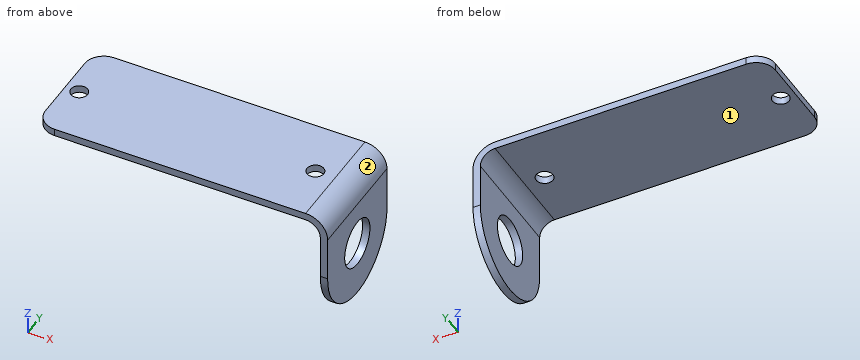
```python
from build123d import *

# Parameters (mm, degrees)
SKETCH1_W                  = 53.93
SKETCH1_H                  = 22.93
BOSS_EXTRUDE1_DEPTH        = 1.5
M3_CLEARANCE_HOLE1_D       = 3.4
M3_CLEARANCE_HOLE1_DEPTH   = 27
M3_CLEARANCE_HOLE1_TIP     = 1.021463052
FILLET1_R                  = 3.9
BOSS_EXTRUDE2_START        = -1.5
SKETCH4_R                  = 4.875
BOSS_EXTRUDE2_DEPTH        = 1.5
SKETCHED_START             = 32.144466887
SKETCHED_BEND1_OUTLINE_W   = 22.93
SKETCHED_BEND1_OUTLINE_H   = 1.5
SKETCHED_BEND1_DEPTH       = 23.855533113
SKETCHED_START_2           = 28.119756887
SKETCHED_BEND1_2_OUTLINE_R = 4.875
SKETCHED_BEND1_2_DEPTH     = 4.5
SKETCHED_START_3           = -11.465
SKETCHED_BEND1_3_DEPTH     = 22.93


with BuildPart() as part:
    # Sketch1 → Boss-Extrude1 (new body)
    with BuildSketch(Plane.XY.offset(1.5)):
        Rectangle(SKETCH1_W, SKETCH1_H)
    extrude(amount=-BOSS_EXTRUDE1_DEPTH)

    # M3 Clearance Hole1
    with Locations(Plane.XY.offset(1.5)):
        with Locations((-24.0755, 0), (24.0755, 0)):
            Hole(M3_CLEARANCE_HOLE1_D / 2, depth=M3_CLEARANCE_HOLE1_DEPTH)
            with Locations((0, 0, -(M3_CLEARANCE_HOLE1_DEPTH + M3_CLEARANCE_HOLE1_TIP / 2))):  # 118° drill point
                Cone(0, M3_CLEARANCE_HOLE1_D / 2, M3_CLEARANCE_HOLE1_TIP, mode=Mode.SUBTRACT)

    # Fillet1
    fillet1_edges = [part.edges().sort_by_distance(p)[0] for p in [
        (-26.965, -11.465, 0.75),
        (-26.965, 11.465, 0.75),
        (26.965, 11.465, 0.75),
        (26.965, -11.465, 0.75),
    ]]
    fillet(fillet1_edges, radius=FILLET1_R)

    # Sketch4 → Boss-Extrude2 (add)
    with BuildSketch(Plane.XY.offset(1.5).offset(BOSS_EXTRUDE2_START)):
        with BuildLine():
            Line((23.065, 11.465), (43.065, 11.465))
            ThreePointArc((43.065, 11.465), (54.53, 0), (43.065, -11.465))
            Line((43.065, -11.465), (23.065, -11.465))
            ThreePointArc((23.065, -11.465), (25.822716447, -10.322716447), (26.965, -7.565))
            Line((26.965, -7.565), (26.965, 7.565))
            ThreePointArc((26.965, 7.565), (25.822716447, 10.322716447), (23.065, 11.465))
        make_face()
        with Locations((43.065, 0)):
            Circle(SKETCH4_R, mode=Mode.SUBTRACT)
    extrude(amount=BOSS_EXTRUDE2_DEPTH)

    # Sketched Bend1: read off the stored shape, not the designer's step
    # Sketched Bend1 outline → Sketched Bend1 (cut)
    with BuildSketch(Plane.YZ.offset(SKETCHED_START)):
        with Locations((0, 0.75)):
            Rectangle(SKETCHED_BEND1_OUTLINE_W, SKETCHED_BEND1_OUTLINE_H)
    extrude(amount=SKETCHED_BEND1_DEPTH, mode=Mode.SUBTRACT)

    # Sketched Bend1 2 outline → Sketched Bend1 2 (add)
    with BuildSketch(Plane.YZ.offset(SKETCHED_START_2)):
        with BuildLine():
            Line((-11.465, 0), (-11.465, -12.054756887))
            ThreePointArc((-11.465, -12.054756887), (0, -23.519756887), (11.465, -12.054756887))
            Line((11.465, -12.054756887), (11.465, 0))
            Line((11.465, 0), (-11.465, 0))
        make_face()
        with Locations((0, -12.054756887)):
            Circle(SKETCHED_BEND1_2_OUTLINE_R, mode=Mode.SUBTRACT)
    extrude(amount=SKETCHED_BEND1_2_DEPTH)

    # Sketched Bend1 3 outline → Sketched Bend1 3 (cut)
    with BuildSketch(Plane(origin=(0, 0, 0), x_dir=(1, 0, 0), z_dir=(0, 1, 0)).offset(SKETCHED_START_3)):
        with BuildLine():
            ThreePointArc((28.119756887, 0), (30.241077231, 0.878679656), (31.119756887, 3))
            Line((31.119756887, 3), (31.119756887, 25))
            Line((31.119756887, 25), (28.119756887, 25))
            Line((28.119756887, 25), (28.119756887, 0))
        make_face()
        with BuildLine():
            Line((32.619756887, 0), (32.619756887, 3))
            ThreePointArc((32.619756887, 3), (31.301737402, -0.181980515), (28.119756887, -1.5))
            Line((28.119756887, -1.5), (27, -1.5))
            Line((27, -1.5), (27, -3))
            Line((27, -3), (32.144466887, -3))
            Line((32.144466887, -3), (32.144466887, 0))
            Line((32.144466887, 0), (32.619756887, 0))
        make_face()
    extrude(amount=SKETCHED_BEND1_3_DEPTH, mode=Mode.SUBTRACT)


solid = part.part
```
Can you work these out from the model? Positions are in its coordinate system, mm. Face numbers are marked on the shaded views. A direction names the side the tool comes from. Give positions to 0.01 mm unless a question says otherwise; leave off trailing zeros. Loops run counter-clockwise (first coordinate to the right, second up) from the corner with the lowest first, then second, coordinate; pieces in that order, holes last. Notation, with made-up numbers: M 57,34.5 L 111,34.5 A11 cw 111,40.5 Z; hole C 20,40.25 d11. An arc over 180 degrees is marked long. Answer in a Markdown table with one row per item.
1. Suppose I cut it at B-B on y = -2.25. Write out the boundary of the cut face in (x, z) (3 decimals).
Taken from the geometry:
| item | result |
|---|---|
| outline | M -26.965,0 L 28.12,0 A3 cw 31.12,-3 L 31.12,-7.73 L 32.62,-7.73 L 32.62,-3 A4.5 ccw 28.12,1.5 L -26.965,1.5 Z; M 31.12,-23.297 L 32.62,-23.297 L 32.62,-16.379 L 31.12,-16.379 Z |
2. Suppose I cut it at A-A on z = -15.75. Write out the boundary of the cut face in (x, y), plus the area to 3 significant figures.
Taken from the geometry:
| item | result |
|---|---|
| outline | M 31.12,-10.85 L 32.62,-10.85 L 32.62,-3.18 L 31.12,-3.18 Z; M 31.12,3.18 L 32.62,3.18 L 32.62,10.85 L 31.12,10.85 Z |
| area | 23.0 mm² |
3. For pin 1 Ø5 at (x, y) = (25, 3.5) entering from -Z; pin 2 Ø10.5 at (y, z) = (2, -17) entering from -X, each with a flat end and sliding along its axis, tell me the tip position at first contact or that it passes through.
Taken from the geometry:
| item | result |
|---|---|
| pin 1 | stops at z = 0 |
| pin 2 | stops at x = 31.12 |
4. If I drill on line 1 along Z through (x, y) = (11, 0.5); line 2 along X through (y, z) = (10.25, -3.5); line 3 along Z through (x, y) = (31.9, 0), over which ranges is the centre line in solid material (lowest first)?
Taken from the geometry:
| item | result |
|---|---|
| line 1 | z = 0 to 1.5 |
| line 2 | x = 31.12 to 32.62 |
| line 3 | z = -23.52 to -16.93, -7.18 to -0.56 |
5. Suppose I cut it at D-D on x = 2. Write out the boundary of the cut face in (y, z) (3 decimals).
Taken from the geometry:
| item | result |
|---|---|
| outline | M -11.465,0 L 11.465,0 L 11.465,1.5 L -11.465,1.5 Z |
6. Which directions (+Z, -Z, +X, -X, +Y, -Y) give clear straight access to the entire face, cutting with the end or side of a thin tool? Please do the marked faces 1 and 2.
Taken from the geometry:
| item | result |
|---|---|
| face 1 | -Z, -X, +Y, -Y |
| face 2 | +Z, +X, +Y, -Y |
7. Suppose I cut it at C-C on y = -6. Write out the boundary of the cut face in (x, z) (3 decimals), plus the area to 3 significant figures.
Taken from the geometry:
| item | result |
|---|---|
| outline | M -26.965,0 L 28.12,0 A3 cw 31.12,-3 L 31.12,-21.824 L 32.62,-21.824 L 32.62,-3 A4.5 ccw 28.12,1.5 L -26.965,1.5 Z |
| area | 120 mm² |
